```python
from build123d import *

# Parameters (mm, degrees)
F0_W     = 11
F0_H     = 9
F0_W_2   = 7
F0_H_2   = 5
F1_DEPTH = 8
F2_W     = 5
F2_H     = 4.881562
F3_DEPTH = 5
F4_R     = 1.75
F5_DEPTH = 2
F6_R     = 1.75
F7_DEPTH = 2
F8_SIZE  = 1
F9_R     = 1


with BuildPart() as f1:
    # F0 (on Front) → F1 (new body)
    with BuildSketch(Plane.XZ):
        Rectangle(F0_W, F0_H)
        Rectangle(F0_W_2, F0_H_2, mode=Mode.SUBTRACT)
    extrude(amount=F1_DEPTH)

    # F2 (on face) → F3 (cut)
    with BuildSketch(Plane.XY.offset(4.5)):
        with Locations((0, -5.559219)):
            Rectangle(F2_W, F2_H)
    extrude(amount=-F3_DEPTH, mode=Mode.SUBTRACT)

    # F4 (on face) → F5 (join)
    with BuildSketch(Plane(origin=(-5.5, 0, 0), x_dir=(0, -1, 0), z_dir=(-1, 0, 0))):
        with Locations((2.55, 0)):
            Circle(F4_R)
    extrude(amount=F5_DEPTH)

    # F6 (on face) → F7 (join)
    with BuildSketch(Plane.YZ.offset(5.5)):
        with Locations((-2.55, 0)):
            Circle(F6_R)
    extrude(amount=F7_DEPTH)

    # F8
    f8_edges = [f1.edges().sort_by_distance(p)[0] for p in [
        (0, -3.118438, 2.5),
    ]]
    chamfer(f8_edges, length=F8_SIZE)

    # F9
    f9_edges = [f1.edges().sort_by_distance(p)[0] for p in [
        (5.5, -4, 4.5),
        (-5.5, -4, 4.5),
        (5.5, -4, -4.5),
        (-5.5, -4, -4.5),
    ]]
    fillet(f9_edges, radius=F9_R)


solid = f1.part
```
Geometry: final body of the model. Coordinates: model frame, mm. A direction names the side the tool comes from. Give positions to 0.01 mm unless a question says otherwise; leave off trailing zeros. Order: outer loops, then holes, each group sorted by start corner. A loop starts at its lowest first (then second) coordinate and runs counter-clockwise, first axis right, second up. Notation, with made-up numbers: M -24,18.5 L 9,18.5 A26 ccw 9,40.5 Z; hole C -2.75,-26 d11. An arc over 180 degrees is marked long. Answer as CSV lines item,"result". Start each with the question number.
1) Cut plane B-B (z = 0). Output: boundary loops of the cut face in (x, y), then the cut area to 3 significant figures.
2) Line query: line 1 (X direction, y = -5, z = 0.25); line 2 (X direction, y = -3.5, z = -0.25); line 3 (Z direction, x = -3, y = -2.25). Output: solid intervals per line, ascending. Write a range as from..to.
3) Cut plane A-A (x = -1). Output: boundary loops of the cut face in (y, z).
4) Set-up query: faces 5 (the flat face through (-3.5, -4, 0)), 6 (the cylindrical face through (-6.49, -0.8, 0.08)), 7 (the flat face through (-7.5, -3, 0)), 8 (the flat face through (0, -8, -3)), 9 (the flat face through (-0.03, -2.63, 3.01)). Return all of +Z, -Z, +X, -X, +Y, -Y with unobstructed straight access to the full face (end or side cutting, diameter ignored); none if empty.
5) Cut plane C-C (y = -1.5). Output: boundary loops of the cut face in (x, z).
6) Cut plane D-D (y = -6). Output: boundary loops of the cut face in (x, z).
7) First-contact query: P1, Ø0.6, axis at y = -5, z = 3, coming from the +X side; P2, Ø0.8, axis at x = -1, z = 4, coming from the -Y side; P3, Ø1, axis at y = -6, z = 3, coming from the -X side. Flat tips, straight axial feed; report the tip coordinate or a pass-through.
8) Mould query, pull axis X, two halves, no side actions, for faces 1 (the flat face through (0, -4, -2.5)), 2 (the cylindrical face through (6.49, -2.93, -1.71)), 3 (the cylindrical face through (-5.199, -4.056, -4.215)), 4 (the cylindrical face through (5.215, -4.056, -4.199)). Classes: +X half, -X half, draft (parallel to the pull), parting line (faces both ways), or undercut.
Findings below:
1,outline,"M -7.5,-4.3 L -5.5,-4.3 L -5.5,-8 L -3.5,-8 L -3.5,0 L -5.5,0 L -5.5,-0.8 L -7.5,-0.8 Z; M 3.5,-8 L 5.5,-8 L 5.5,-4.3 L 7.5,-4.3 L 7.5,-0.8 L 5.5,-0.8 L 5.5,0 L 3.5,0 Z"
1,area,"46.0 mm²"
2,line 1,"x = -5.5..-3.5, 3.5..5.5"
2,line 2,"x = -7.5..-3.5, 3.5..7.5"
2,line 3,"z = -4.5..-2.5, 2.5..4.5"
3,outline,"M -8,-4.5 L 0,-4.5 L 0,-2.5 L -8,-2.5 Z; M -3.12,3.5 L -2.12,2.5 L 0,2.5 L 0,4.5 L -3.12,4.5 Z"
4,face 5,"+Y, -Y"
4,face 6,"-X"
4,face 7,"+Z, -Z, -X, +Y, -Y"
4,face 8,"+Z, -Z, +X, -X, -Y"
4,face 9,"-Y"
5,outline,"M -7.5,-1.4 L -5.5,-1.4 L -5.5,-3.5 A1 ccw -4.5,-4.5 L 4.5,-4.5 A1 ccw 5.5,-3.5 L 5.5,-1.4 L 7.5,-1.4 L 7.5,1.4 L 5.5,1.4 L 5.5,3.5 A1 ccw 4.5,4.5 L -4.5,4.5 A1 ccw -5.5,3.5 L -5.5,1.4 L -7.5,1.4 Z; hole M -3.5,-2.5 L 3.5,-2.5 L 3.5,2.5 L -3.5,2.5 Z"
6,outline,"M -5.5,-3.5 A1 ccw -4.5,-4.5 L 4.5,-4.5 A1 ccw 5.5,-3.5 L 5.5,3.5 A1 ccw 4.5,4.5 L 2.5,4.5 L 2.5,2.5 L 3.5,2.5 L 3.5,-2.5 L -3.5,-2.5 L -3.5,2.5 L -2.5,2.5 L -2.5,4.5 L -4.5,4.5 A1 ccw -5.5,3.5 Z"
7,P1,"stops at x = 5.5"
7,P2,"stops at y = -3.12"
7,P3,"stops at x = -5.5"
8,face 1,"undercut"
8,face 2,"draft"
8,face 3,"-X half"
8,face 4,"+X half"
